Design review of the part built by this model. Coordinates are the model's own, in mm. A direction names the side the tool comes from. Coordinates: 2 decimals unless noted, no trailing zeros. Loops run counter-clockwise (first coordinate to the right, second up) from the corner with the lowest first, then second, coordinate; pieces in that order, holes last. Notation, with made-up numbers: M 47,49.5 L 58,49.5 A23 ccw 58,71.5 Z; hole C 87,6.25 d7. An arc over 180 degrees is marked long. Put each result on its own line as item: value. Start each with the question number.
(1) Take a section at D-D, the plane x = 2.75. Give the boundary of the cut face in (y, z), then the cut area to 3 significant figures.
(2) For probe 1 along Y at (x, z) = (21, 2.7); probe 2 along Y at (x, z) = (11.1, 0.65); probe 3 along Y at (x, z) = (4.5, 1.2), list the stretches that pass through material, from the lowest coordinate up. Write a range as [from, to].
(3) Take a section at A-A, the plane y = 4. Give the boundary of the cut face in (x, z).
(4) The part is to be moulded in two halves that separate along Y. For faces 6 (the flat face through (22, 12.5, 1)), 7 (the flat face through (10, 13, 0)), 8 (the flat face through (10, 23.5, 1)), say which applies: +Y half, -Y half, draft (parallel to the pull), parting line (faces both ways), or undercut.
(5) Take a section at C-C, the plane x = 11.1. Give the boundary of the cut face in (y, z).
(6) Clearance check with flat-ended pins moving along their axes: pin 1 (0.9 mm diameter, centred on x = 21.5, z = 1, fed in from -Y); pin 2 (1.5 mm diameter, centred on y = 2.5, z = 1.5, fed in from -X); pin 3 (1.5 mm diameter, centred on y = 11.5, z = 2, fed in from -X). State where each tip first meets the part, or that it passes through.
(7) Take a section at B-B, the plane z = 2.15. Give the boundary of the cut face in (x, y), then the cut area to 3 significant figures.
(8) For faces 1 (the flat face through (3, 8, 2)), 2 (the flat face through (22, 3, 1)), 3 (the flat face through (22, 8, 1)), 4 (the flat face through (14.1, 22, 1)), 5 (the flat face through (3, 20.5, 1)), list the 3-axis set-ups (+Z, -Z, +X, -X, +Y, -Y) from which the entire face can be reached by the end or side of a thin tool; tool diameter is ignored.
```python
from build123d import *

# Parameters (mm, degrees)
BASE_DEPTH            = 3
ESBO_O1_R             = 4.25
PASSAGEMLEDELDR_DEPTH = 3


with BuildPart() as part:
    # BaseEsboco → Base (new body)
    with BuildSketch(Plane.XY):
        Polygon((0, 0), (6, 0), (6, -3), (14.1, -3), (14.1, 0), (20.1, 0), (20.1, 3), (23.1, 3), (23.1, 8), (20.1, 8), (20.1, 12.5), (23.1, 12.5), (23.1, 17.5), (20.1, 17.5), (20.1, 20.5), (14.1, 20.5), (14.1, 23.5), (6, 23.5), (6, 20.5), (0, 20.5), (0, 17.5), (-3, 17.5), (-3, 12.5), (0, 12.5), (0, 8), (-3, 8), (-3, 3), (0, 3), align=None)
    extrude(amount=BASE_DEPTH)

    # Esboço1 → PassagemLEDeLDR (cut)
    with BuildSketch(Plane.XY.offset(3)):
        with Locations((11.1, 4)):
            Circle(ESBO_O1_R)
        Polygon((0, 8), (6, 8), (6, 0), (0, 0), (0, 3), (-3, 3), (-3, 8), align=None)
    extrude(amount=-PASSAGEMLEDELDR_DEPTH, mode=Mode.SUBTRACT)


solid = part.part
```
Computed values:
1. outline: M 8,0 L 20.5,0 L 20.5,3 L 8,3 Z
1. area: 37.5 mm^2
2. probe 1: y = [3, 8], [12.5, 17.5]
2. probe 2: y = [-3, -0.25], [8.25, 23.5]
2. probe 3: y = [8, 20.5]
3. outline: M 6,0 L 6.85,0 L 6.85,3 L 6,3 Z; M 15.35,0 L 23.1,0 L 23.1,3 L 15.35,3 Z
4. face 6: undercut
4. face 7: draft
4. face 8: +Y half
5. outline: M -3,0 L -0.25,0 L -0.25,3 L -3,3 Z; M 8.25,0 L 23.5,0 L 23.5,3 L 8.25,3 Z
6. pin 1: stops at y = 3
6. pin 2: stops at x = 6
6. pin 3: stops at x = 0
7. outline: M -3,12.5 L 0,12.5 L 0,8 L 6,8 L 6,-3 L 14.1,-3 L 14.1,0 L 20.1,0 L 20.1,3 L 23.1,3 L 23.1,8 L 20.1,8 L 20.1,12.5 L 23.1,12.5 L 23.1,17.5 L 20.1,17.5 L 20.1,20.5 L 14.1,20.5 L 14.1,23.5 L 6,23.5 L 6,20.5 L 0,20.5 L 0,17.5 L -3,17.5 Z; hole C 11.1,4 d8.5
7. area: 401 mm^2
8. face 1: +Z, -Z, -X, -Y
8. face 2: +Z, -Z, +X, -Y
8. face 3: +Z, -Z, +X
8. face 4: +Z, -Z, +X, +Y
8. face 5: +Z, -Z, -X, +Y
